The listing builds one solid part. Answer for the finished solid, in the listing's coordinates (mm). A direction names the side the tool comes from. Coordinates: 2 decimals unless noted, no trailing zeros. Answer as CSV lines item,"result".
Autodesk Inventor part; units mm, degrees
ref_plane "YZ Plane" through (0, 0, 0) normal (1, 0, 0) x (0, 1, 0)
ref_plane "XZ Plane" through (0, 0, 0) normal (0, 1, 0) x (-1, 0, 0)
ref_plane "XY Plane" through (0, 0, 0) normal (0, 0, 1) x (1, 0, 0)
sketch "T-Slot 4040 Base" plane through (0, 0, 0) normal (0, 0, 1) x (1, 0, 0)
  line L0 (-28, 0) -> (28, 0) construction
  line L1 (0, -28) -> (0, 28) construction
  circle A0 centre (0, 0) radius 5.1
  line L2 (-7.5, -7.5) -> (7.5, -7.5)
  line L3 (7.5, -7.5) -> (7.5, 7.5)
  line L4 (7.5, 7.5) -> (-7.5, 7.5)
  line L5 (-7.5, 7.5) -> (-7.5, -7.5)
  line L6 (-7.5, -7.5) -> (7.5, 7.5) construction
  line L7 (7.5, -7.5) -> (-7.5, 7.5) construction
  line L8 (-20, 20) -> (20, 20)
  line L9 (20, 20) -> (20, -20)
  line L10 (20, -20) -> (-20, -20)
  line L11 (-20, -20) -> (-20, 20)
  line L12 (-20, 20) -> (20, -20) construction
  line L13 (20, 20) -> (-20, -20) construction
  line L14 (20, 5) -> (14.5, 5)
  line L15 (14.5, 5) -> (14.5, 10)
  line L16 (14.5, 10) -> (12.4749, 10)
  line L17 (12.4749, 10) -> (7.5, 5.0251)
  line L18 (5, 20) -> (5, 14.5)
  line L19 (5, 14.5) -> (10, 14.5)
  line L20 (10, 14.5) -> (10, 12.4749)
  line L21 (10, 12.4749) -> (5.0251, 7.5)
  line L22 (18.5, 18.5) -> (11.5, 18.5)
  line L23 (11.5, 18.5) -> (11.5, 11.5)
  line L24 (11.5, 11.5) -> (18.5, 11.5)
  line L25 (18.5, 11.5) -> (18.5, 18.5)
  line L26 (18.5, 18.5) -> (11.5, 11.5) construction
  line L27 (11.5, 18.5) -> (18.5, 11.5) construction
  line L28 (3.0732, 1.3088) -> (4.38, 2.6125) construction
  line L29 (5.905, 4.1338) -> (4.1393, 5.9037)
  line L30 (4.1393, 5.9037) -> (2.6122, 4.3802)
  line L31 (1.3075, 3.0787) -> (3.0732, 1.3088) construction
  line L32 (3.0732, 1.3088) -> (4.1393, 5.9037) construction
  line L33 (5.905, 4.1338) -> (1.3075, 3.0787) construction
  line L34 (4.38, 2.6125) -> (5.905, 4.1338)
  line L35 (2.6122, 4.3802) -> (1.3075, 3.0787) construction
  line L36 (-20, 5) -> (-14.5, 5)
  line L37 (-14.5, 5) -> (-14.5, 10)
  line L38 (-14.5, 10) -> (-12.4749, 10)
  line L39 (-12.4749, 10) -> (-7.5, 5.0251)
  line L40 (-5, 20) -> (-5, 14.5)
  line L41 (-5, 14.5) -> (-10, 14.5)
  line L42 (-10, 14.5) -> (-10, 12.4749)
  line L43 (-10, 12.4749) -> (-5.0251, 7.5)
  line L44 (-18.5, 18.5) -> (-11.5, 18.5)
  line L45 (-11.5, 18.5) -> (-11.5, 11.5)
  line L46 (-11.5, 11.5) -> (-18.5, 11.5)
  line L47 (-18.5, 11.5) -> (-18.5, 18.5)
  line L48 (-5.905, 4.1338) -> (-4.1393, 5.9037)
  line L49 (-4.1393, 5.9037) -> (-2.6122, 4.3802)
  line L50 (-4.38, 2.6125) -> (-5.905, 4.1338)
  line L51 (7.5, -7.5) -> (-7.5, -7.5)
  line L52 (20, -5) -> (14.5, -5)
  line L53 (14.5, -5) -> (14.5, -10)
  line L54 (14.5, -10) -> (12.4749, -10)
  line L55 (12.4749, -10) -> (7.5, -5.0251)
  line L56 (5, -20) -> (5, -14.5)
  line L57 (5, -14.5) -> (10, -14.5)
  line L58 (10, -14.5) -> (10, -12.4749)
  line L59 (10, -12.4749) -> (5.0251, -7.5)
  line L60 (18.5, -18.5) -> (11.5, -18.5)
  line L61 (11.5, -18.5) -> (11.5, -11.5)
  line L62 (11.5, -11.5) -> (18.5, -11.5)
  line L63 (18.5, -11.5) -> (18.5, -18.5)
  line L64 (18.5, -18.5) -> (11.5, -11.5) construction
  line L65 (11.5, -18.5) -> (18.5, -11.5) construction
  line L66 (3.0732, -1.3088) -> (4.38, -2.6125) construction
  line L67 (5.905, -4.1338) -> (4.1393, -5.9037)
  line L68 (4.1393, -5.9037) -> (2.6122, -4.3802)
  line L69 (1.3075, -3.0787) -> (3.0732, -1.3088) construction
  line L70 (3.0732, -1.3088) -> (4.1393, -5.9037) construction
  line L71 (5.905, -4.1338) -> (1.3075, -3.0787) construction
  line L72 (4.38, -2.6125) -> (5.905, -4.1338)
  line L73 (2.6122, -4.3802) -> (1.3075, -3.0787) construction
  line L74 (-4.38, -2.6125) -> (-5.905, -4.1338)
  line L75 (-4.1393, -5.9037) -> (-2.6122, -4.3802)
  line L76 (-5.905, -4.1338) -> (-4.1393, -5.9037)
  line L77 (-12.4749, -10) -> (-7.5, -5.0251)
  line L78 (-10, -12.4749) -> (-5.0251, -7.5)
  line L79 (-10, -14.5) -> (-10, -12.4749)
  line L80 (-5, -14.5) -> (-10, -14.5)
  line L81 (-5, -20) -> (-5, -14.5)
  line L82 (-18.5, -18.5) -> (-11.5, -18.5)
  line L83 (-11.5, -18.5) -> (-11.5, -11.5)
  line L84 (-11.5, -11.5) -> (-18.5, -11.5)
  line L85 (-18.5, -11.5) -> (-18.5, -18.5)
  line L86 (-14.5, -10) -> (-12.4749, -10)
  line L87 (-14.5, -5) -> (-14.5, -10)
  line L88 (-20, -5) -> (-14.5, -5)
  point P0 (15, 15)
  point P1 (3.6062, 3.6062)
  point P2 (3.6062, 3.6062)
  point P3 (15, -15)
  point P4 (3.6062, -3.6062)
  point P5 (3.6062, -3.6062)
  dimension "d9" = 10.2
  dimension "d12" = 40
  dimension "d13" = 40
  dimension "d14" = 5.5
  dimension "d15" = 15
  dimension "d16" = 7
  dimension "d17" = 10
  dimension "d20" = 1.75
  dimension "d21" = 7
  dimension "d22" = 2
  dimension "d29" = 1.5
  dimension "d30" = 2.5
extrude "Extrusion1" add sketch "T-Slot 4040 Base" along normal blind 640 contours L5 L4 L3 L2 | L2 L78 L79 L80 L81 L10 L11 L88 L87 L86 L77 L5 | L2 L3 L55 L54 L53 L52 L9 L10 L56 L57 L58 L59 | L39 L38 L37 L36 L11 L8 L40 L41 L42 L43 L4 L5 | L3 L4 L21 L20 L19 L18 L8 L9 L14 L15 L16 L17
fillet "Rundung1" radius 1 16 edges at (11.5, 18.5, 320) (18.5, 18.5, 320) (18.5, 11.5, 320) (11.5, 11.5, 320) (-11.5, 18.5, 320) (-18.5, 18.5, 320) (-18.5, 11.5, 320) (-11.5, 11.5, 320) (-18.5, -11.5, 320) (-11.5, -11.5, 320) (-11.5, -18.5, 320) (-18.5, -18.5, 320) (11.5, -18.5, 320) (11.5, -11.5, 320) (18.5, -11.5, 320) (18.5, -18.5, 320)
fillet "Rundung2" radius 3 4 edges at (20, 20, 320) (20, -20, 320) (-20, -20, 320) (-20, 20, 320)
properties part number "T-SLOT 4040 B-Type 640mm"
Q1. The mould has two halves that part along X. Classify faces 1 (the flat face through (20, -11, 316)), 2 (the flat face through (-20, 11, 316)), 3 (the flat face through (0, 7.5, 316)): pulls with the +X half, pulls with the -X half, needs draft (parallel to the pull), parting line crosses it, or undercut.
Output:
face 1,"pulls with the +X half"
face 2,"pulls with the -X half"
face 3,"undercut"
Q2. Straight lines are drawn through the part: line 1 (Y direction, x = -13, z = 180.5); line 2 (Y direction, x = -16.5, z = 609.5). For each, find the intervals that lie inside material, in ascending order.
Output:
line 1,"-20 to -18.5, -11.5 to -10, 10 to 11.5, 18.5 to 20"
line 2,"-20 to -18.5, -11.5 to -5, 5 to 11.5, 18.5 to 20"
Q3. For faces 4 (the flat face through (-7.5, 0, 316)), 5 (the flat face through (-11, 20, 316)), 6 (the flat face through (0, -7.5, 316)), 7 (the flat face through (-20, -11, 316)), 8 (the flat face through (7.5, 0, 316)), determine the directions among +Z, -Z, +X, -X, +Y, -Y from which every point of the face is accessible in a straight line to the end or side of a thin tool.
Output:
face 4,"+Z, -Z, -X"
face 5,"+Z, -Z, +X, -X, +Y"
face 6,"+Z, -Z, -Y"
face 7,"+Z, -Z, -X, +Y, -Y"
face 8,"+Z, -Z, +X"
Q4. Flat-ended cylindrical pins translate along their axes: pin 1 Ø1.6 at (x, z) = (-18, 301.5) entering from +Y; pin 2 Ø3 at (x, z) = (-2.5, 423) entering from +Y; pin 3 Ø5 at (x, z) = (0.5, 178.5) entering from -Y. Find the tip coordinate at first contact, or state that the pin passes through.
Output:
pin 1,"y = 19.99"
pin 2,"y = 7.5"
pin 3,"y = -7.5"
Q5. Find section A-A (z = 180.5). Count the separate pieces of the cut face and the enclosed holes in it, and give its area (3 significant figures).
Output:
separate pieces,"1"
enclosed holes,"5"
area,"616 mm2"
